Solid Edge part; units mm, degrees
sketch "Sketch1" plane through (0, 0, 0) normal (0, -1, 0) x (1, 0, 0)
  circle A0 centre (0, 51) radius 3.15
  line L0 (25, 0) -> (12.5, 51)
  line L1 (0, 0) -> (25, 0)
  line L2 (0, 0) -> (-25, 0)
  line L3 (-25, 0) -> (-12.5, 50.9918)
  arc A1 (-12.5, 50.9918) -> (12.5, 51) centre (0, 51) cw
extrude "Protrusion1" add sketch "Sketch1" against normal blind 10
sketch "Sketch2" plane through (0, 10, 31.75) normal (0, 1, 0) x (-1, 0, 0)
  line L0 (23.5292, -25.75) -> (-23.5294, -25.75)
  line L1 (-23.5294, -25.75) -> (-25, -31.75)
  line L2 (-25, -31.75) -> (25, -31.75)
  line L3 (25, -31.75) -> (23.5292, -25.75)
extrude "ExtrudedProtrusion_5" add sketch "Sketch2" along normal blind 15
sketch "Sketch3" plane through (0.0001, 17.5, 6) normal (0, 0, 1) x (-1, 0, 0)
  line L0 (3.0001, 7.5) -> (3.0001, -7.5)
  line L1 (3.0001, -7.5) -> (-2.9999, -7.5)
  line L2 (-2.9999, -7.5) -> (-2.9999, 7.5)
  line L3 (-2.9999, 7.5) -> (3.0001, 7.5)
extrude "ExtrudedProtrusion_6" add sketch "Sketch3" along normal blind 5
chamfer "Chamfer_4" distance 5 angle 45 2 edges at (0, 10, 11) (0, 25, 11)
chamfer "Chamfer_5" distance 3 angle 45 2 edges at (3, 10, 11) (-3, 10, 11)
sketch "Sketch4" plane through (13.2647, 17.5, 6) normal (0, 0, 1) x (0, 1, 0)
  circle A0 centre (0, 0) radius 2.5
  circle A1 centre (0, 26.5293) radius 2.5
extrude "Cutout1" cut sketch "Sketch4" against normal up to next
Source: CAD feature listing. Evaluate the final solid. Frame: model axes, mm. A direction names the side the tool comes from. Coordinates: 2 decimals unless noted, no trailing zeros. Loops run counter-clockwise (first coordinate to the right, second up) from the corner with the lowest first, then second, coordinate; pieces in that order, holes last. Notation, with made-up numbers: (12, 8.25) -> (70, 8.25) arc R15 cw to (70, 26.25) -> close; hole circle Ø3 at (44, 87). An arc over 180 degrees is marked (long way). Answer in a Markdown table with one row per item. Add a question column.
Q1. Section D-D on z = 23. Return the cut outline in (x, y), and give its area (3 significant figures).
Q2. Section C-C on y = 14. Return the cut outline in (x, z).
Q3. Section B-B on x = 0. Return the cut outline in (y, z).
Q4. Section A-A on y = 17.5. Return the cut outline in (x, z), and give its area (3 significant figures).
Q5. Contact query for flat-ended pins moving along their axis: pin 1 Ø4 at (y, z) = (17, 9.5) entering from -X; pin 2 Ø8 at (x, y) = (10, 17) entering from +Z; pin 3 Ø6.5 at (x, y) = (13.26, 17.5) entering from -Z; pin 4 Ø6 at (x, z) = (-2, 44.5) entering from +Y. Output: stop coordinate, or through.
Q6. Pull-direction query (Y, two-part tool) for faces 1 (the face through (13.2, 15, 3)), 2 (the face through (1, 10, 32)), 3 (the face through (-16, 19, 6)); classes: pulls with the +Y half, pulls with the -Y half, needs draft (parallel to the pull), parting line crosses it, or undercut.
Q7. Ray query, line 1 along X through (y, z) = (17.5, 3.55); line 2 along X through (y, z) = (17.5, 1.65); line 3 along Z through (x, y) = (0, 3.25). Return the intervals inside material, ascending.
Q8. Reachability of faces 4 (the face through (3, 18, 8)), 5 (the face through (-4, 12, 10)), 6 (the face through (0, 18, 11)), 7 (the face through (-0.683, 4.93, 47.925)) from +Z, -Z, +X, -X, +Y, -Y: full face, straight path, thin tool, end or side. Return the list, or none.
Computed values:
| question | item | result |
|---|---|---|
| 1 | outline | (-19.36, 0) -> (19.36, 0) -> (19.36, 10) -> (-19.36, 10) -> close |
| 1 | area | 387 mm^2 |
| 2 | outline | (-25, 0) -> (25, 0) -> (23.53, 6) -> (3, 6) -> (3, 12) -> (-3, 12) -> (-3, 6) -> (-23.53, 6) -> close |
| 3 | outline | (0, 0) -> (25, 0) -> (25, 6) -> (20, 11) -> (15, 11) -> (10, 16) -> (10, 47.85) -> (0, 47.85) -> close; (0, 54.15) -> (10, 54.15) -> (10, 63.5) -> (0, 63.5) -> close |
| 4 | outline | (-25, 0) -> (-15.76, 0) -> (-15.76, 6) -> (-23.53, 6) -> close; (-10.76, 0) -> (10.76, 0) -> (10.76, 6) -> (3, 6) -> (3, 11) -> (-3, 11) -> (-3, 6) -> (-10.76, 6) -> close; (15.76, 0) -> (25, 0) -> (23.53, 6) -> (15.76, 6) -> close |
| 4 | area | 261 mm^2 |
| 5 | pin 1 | stops at x = -3 |
| 5 | pin 2 | stops at z = 6 |
| 5 | pin 3 | stops at z = 0 |
| 5 | pin 4 | stops at y = 10 |
| 6 | face 1 | undercut |
| 6 | face 2 | pulls with the +Y half |
| 6 | face 3 | needs draft |
| 7 | line 1 | x = -24.13 to -15.76, -10.76 to 10.76, 15.76 to 24.13 |
| 7 | line 2 | x = -24.6 to -15.76, -10.76 to 10.76, 15.76 to 24.6 |
| 7 | line 3 | z = 0 to 47.85, 54.15 to 63.5 |
| 8 | face 4 | +Z, +X, +Y |
| 8 | face 5 | +Z, -X, +Y |
| 8 | face 6 | +Z, +X, -X, +Y |
| 8 | face 7 | +Y, -Y |
